CAD build for the part. Positions are in the model's coordinates, mm. Coordinates: 2 decimals unless noted, no trailing zeros. Order: outer loops, then holes, each group sorted by start corner. A loop starts at its lowest first (then second) coordinate and runs counter-clockwise, first axis right, second up. Notation, with made-up numbers: (84.5, -39.5) - (101.5, -39.5) arc R13 cw to (101.5, -26.5) - close; hole circle Ø6 at (42.25, 0.25). An arc over 180 degrees is marked (long way). Use one line per item in the form item = value.
```python
from build123d import *

# Parameters (mm, degrees)
BOSS_EXTRUDE1_DEPTH = 2


with BuildPart() as part:
    # Sketch1 → Boss-Extrude1 (new body)
    with BuildSketch(Plane(origin=(0, 0, 0), x_dir=(1, 0, 0), z_dir=(0, 1, 0))):
        with BuildLine():
            Line((-30, 0), (-30, -35.56))
            Line((-30, -35.56), (30, -35.56))
            Line((30, -35.56), (30, 0))
            ThreePointArc((30, 0), (0, 30), (-30, 0))
        make_face()
        with BuildLine():
            Line((12.336270574, -11.418953413), (-12.336270574, -11.418953413))
            ThreePointArc((-12.336270574, -11.418953413), (-23.755223987, 0), (-12.336270574, 11.418953413))
            Line((-12.336270574, 11.418953413), (12.336270574, 11.418953413))
            ThreePointArc((12.336270574, 11.418953413), (23.755223987, 0), (12.336270574, -11.418953413))
        make_face(mode=Mode.SUBTRACT)
    extrude(amount=BOSS_EXTRUDE1_DEPTH)


solid = part.part
```
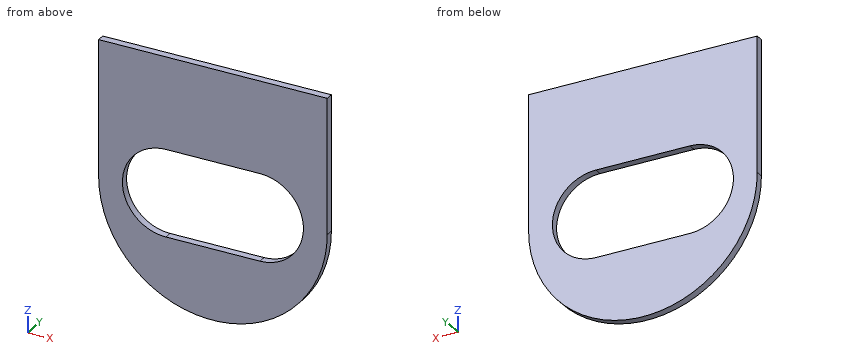
Item 1: Cut at C-C, the plane z = 6.5. Write the cut outline in (x, y), plus the area to 3 significant figures.
Derived:
outline = (-30, 0) - (-21.72, 0) - (-21.72, 2) - (-30, 2) - close; (21.72, 0) - (30, 0) - (30, 2) - (21.72, 2) - close
area = 33.1 mm²
Item 2: Cut at D-D, the plane z = -15.5. Write the cut outline in (x, y).
Derived:
outline = (-25.69, 0) - (25.69, 0) - (25.69, 2) - (-25.69, 2) - close
Item 3: Drill centre lines: line 1 (Z direction, x = -22.5, y = 0.25); line 2 (Z direction, x = 19.5, y = 1.4); line 3 (X direction, y = 0.5, z = -3). Where is each one in solid material? Low to high. Write a range as [from, to].
Derived:
line_1 = [-19.84, -5.2], [5.2, 35.56]
line_2 = [-22.8, -8.89], [8.89, 35.56]
line_3 = [-29.85, -23.35], [23.35, 29.85]
Item 4: Cut at A-A, the plane x = 0. Write the cut outline in (y, z), plus the area to 3 significant figures.
Derived:
outline = (0, -30) - (2, -30) - (2, -11.42) - (0, -11.42) - close; (0, 11.42) - (2, 11.42) - (2, 35.56) - (0, 35.56) - close
area = 85.4 mm²
Item 5: Cut at B-B, the plane y = 0.5. Write the cut outline in (x, z).
Derived:
outline = (-30, 0) arc R30 ccw to (30, 0) - (30, 35.56) - (-30, 35.56) - close; hole (-12.34, -11.42) - (12.34, -11.42) arc R11.42 ccw to (12.34, 11.42) - (-12.34, 11.42) arc R11.42 ccw to start
Item 6: Drop a flat-ended pin along its axis: pin 1 (8 mm diameter, centred on x = 5, z = -5, fed in from -Y). Give the stop position or say it passes through.
Derived:
pin_1 = through
